The figure shows three views and two pictorial views of one solid part (mm, origin at its lowest corner). Answer the questions. A direction names the side the tool comes from. Coordinates: 2 decimals unless noted, no trailing zeros. Loops run counter-clockwise (first coordinate to the right, second up) from the corner with the lowest first, then second, coordinate; pieces in that order, holes last. Notation, with made-up numbers: (37.5, 78.25) -> (41.5, 78.25) arc R30 cw to (41.5, 114.25) -> close; hole circle Ø10 at (18, 82.25). An arc over 180 degrees is marked (long way). Answer as a JSON object with one key per item and string values. Group by question number.
1) Determine the mould class of the marked faces 1, 2 and 3 for opening direction X: released by +X, released by -X, zero draft, split by the parting line, or undercut.
2) Which of the six approach directions +Z, -Z, +X, -X, +Y, -Y give full straight-line access (tool end or side, diameter ignored) to the marked faces 4 and 5?
3) Consider probe 1 along X at (y, z) = (67, 43); probe 2 along Z at (x, y) = (52.5, 5); probe 3 along X at (y, z) = (54, 9). Determine where each line is inside the solid, lowest interval first. Write a range as [from, to].
4) Section C-C, the plane x = 104 is taken. Give the vertices of the cut face in (y, z), plus the area to 3 significant figures.
5) Section D-D, the plane z = 97 is taken. Give the vertices of the cut face in (x, y), plus the area to 3 significant figures.
6) Flat-ended cylindrical pins translate along their axes: P1, Ø3, axis at x = 91.5, y = 26.5, coming from the +Z side; P2, Ø10, axis at x = 25.5, z = 65.5, coming from the +Y side; P3, Ø1.5, axis at y = 57.5, z = 65, coming from the -X side; P4, Ø12.5, axis at y = 74, z = 38.5, coming from the -X side. Find the tip coordinate at first contact, or state that the pin passes through.
7) Section B-B, the plane y = 12 is taken. Give the vertices of the cut face in (x, z) (1 decimal), plus the area to 3 significant figures.
8) Section A-A, the plane z = 16.5 is taken. Give the vertices of the cut face in (x, y), plus the area to 3 significant figures.
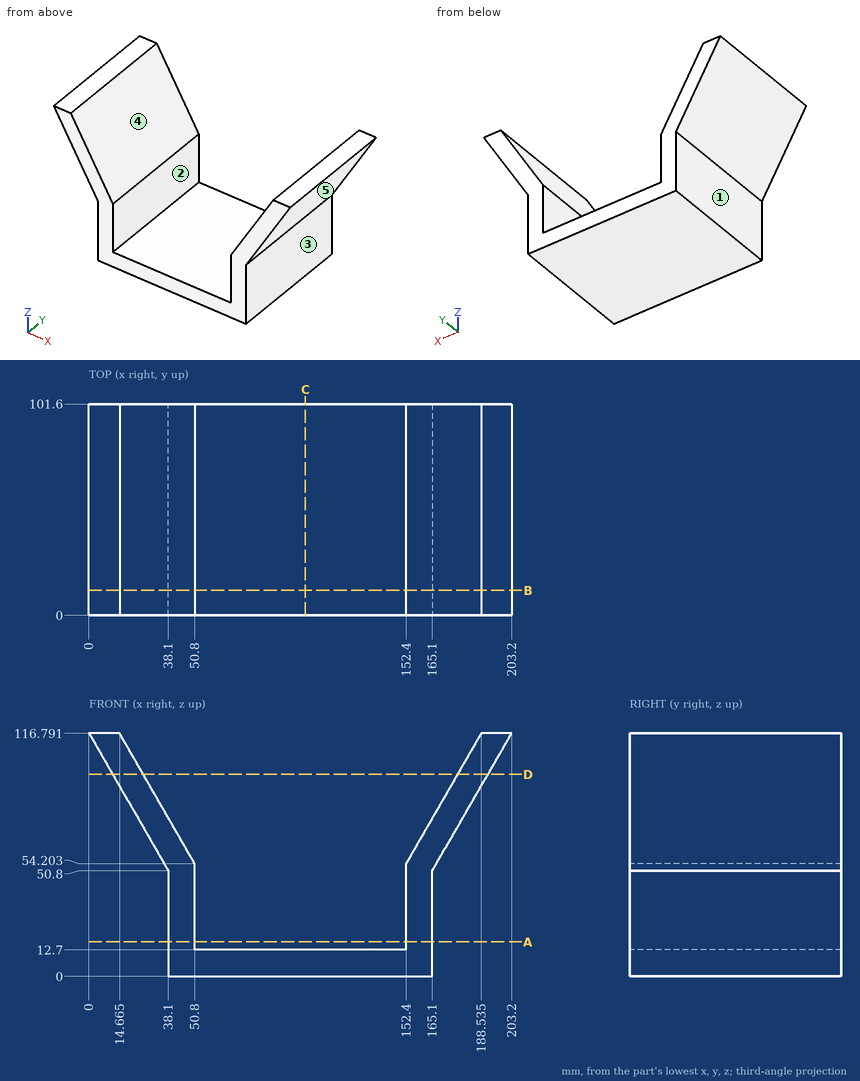
Determined:
{
 "1": {"face 1": "released by -X", "face 2": "undercut", "face 3": "released by +X"},
 "2": {"face 4": "+Z, +Y, -Y", "face 5": "-Z, +X, +Y, -Y"},
 "3": {"probe 1": "[38.1, 50.8], [152.4, 165.1]", "probe 2": "[0, 12.7]", "probe 3": "[38.1, 165.1]"},
 "4": {"outline": "(0, 0) -> (101.6, 0) -> (101.6, 12.7) -> (0, 12.7) -> close", "area": "1,290 mm²"},
 "5": {"outline": "(11.43, 0) -> (26.09, 0) -> (26.09, 101.6) -> (11.43, 101.6) -> close; (177.11, 0) -> (191.77, 0) -> (191.77, 101.6) -> (177.11, 101.6) -> close", "area": "2,980 mm²"},
 "6": {"P1": "z = 12.7", "P2": "y = 101.6", "P3": "x = 29.47", "P4": "x = 38.1"},
 "7": {"outline": "(0, 116.8) -> (38.1, 50.8) -> (38.1, 0) -> (165.1, 0) -> (165.1, 50.8) -> (203.2, 116.8) -> (188.5, 116.8) -> (152.4, 54.2) -> (152.4, 12.7) -> (50.8, 12.7) -> (50.8, 54.2) -> (14.7, 116.8) -> close", "area": "4,510 mm²"},
 "8": {"outline": "(38.1, 0) -> (50.8, 0) -> (50.8, 101.6) -> (38.1, 101.6) -> close; (152.4, 0) -> (165.1, 0) -> (165.1, 101.6) -> (152.4, 101.6) -> close", "area": "2,580 mm²"}
}
